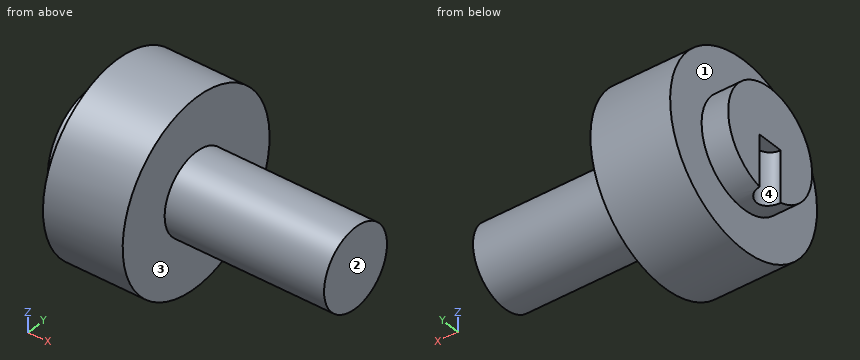
from build123d import *

# Parameters (mm, degrees)
SKETCH_2_R          = 5
CUT_EXTRUDE_1_DEPTH = 20


with BuildPart() as part:
    # Эскиз1 → Повернуть1 (revolve)
    with BuildSketch(Plane.XY, mode=Mode.PRIVATE) as revolve_1_sk:
        Polygon((0, 0), (100, 0), (100, 15), (40, 15), (40, 35), (10, 35), (10, 20), (0, 20), align=None)
    revolve(revolve_1_sk.sketch.rotate(Axis((0, 0, 0), (1, 0, 0)), 90), axis=Axis((0, 0, 0), (1, 0, 0)))

    # Эскиз2 → Вырез-Вытянуть1 (cut)
    with BuildSketch(Plane.XY):
        Circle(SKETCH_2_R)
    extrude(amount=-CUT_EXTRUDE_1_DEPTH, mode=Mode.SUBTRACT)


solid = part.part
CAD build for the part. Positions are in the model's coordinates, mm. Face numbers are marked on the shaded views. A direction names the side the tool comes from. Give positions to 0.01 mm unless a question says otherwise; leave off trailing zeros. Order: outer loops, then holes, each group sorted by start corner. A loop starts at its lowest first (then second) coordinate and runs counter-clockwise, first axis right, second up. Notation, with made-up numbers: (-17, 76) - (36, 76) arc R12 cw to (36, 99) - close; hole circle Ø2 at (63.25, -9.5). An arc over 180 degrees is marked (long way). Write each question's results on one line, items separated by ' | '.
1. Saw through at C-C on x = 25. List the corners of the cut face in (y, z), and give its area (3 significant figures).
Calculated:
outline: circle Ø70 at (0, 0) | area: 3,850 mm2
2. Pin check, flat tips, straight feed: pin 1 (5 mm diameter, centred on y = -27.5, z = -19, fed in from -X); pin 2 (5.5 mm diameter, centred on x = 2, y = 1.5, fed in from -Z); pin 3 (8 mm diameter, centred on x = 33.5, z = 21, fed in from +Y). Stop position of each tip, or through.
Calculated:
pin 1: stops at x = 10 | pin 2: stops at z = -19.94 | pin 3: stops at y = 30.59
3. Saw through at A-A on y = 0. List the corners of the cut face in (x, z).
Calculated:
outline: (0, 0) - (5, 0) - (5, -20) - (10, -20) - (10, -35) - (40, -35) - (40, -15) - (100, -15) - (100, 15) - (40, 15) - (40, 35) - (10, 35) - (10, 20) - (0, 20) - close
4. Saw through at B-B on z = -12. List the corners of the cut face in (x, y), and give its area (3 significant figures).
Calculated:
outline: (0, -16) - (10, -16) - (10, -32.88) - (40, -32.88) - (40, -9) - (100, -9) - (100, 9) - (40, 9) - (40, 32.88) - (10, 32.88) - (10, 16) - (0, 16) - (0, 5) arc R5 cw to (0, -5) - close | area: 3,330 mm2
5. Probe L1, parallel to X at y = -18.5, z = 14; L2, parallel to X at y = -10, z = -12; L3, parallel to Z at x = 57, y = 5.5. List the from-to ranges inside material, lowest first. Write a range as from..to.
Calculated:
L1: x = 10..40 | L2: x = 0..40 | L3: z = -13.96..13.96
6. Saw through at D-D on y = -11. List the corners of the cut face in (x, z), and give its area (3 significant figures).
Calculated:
outline: (0, -16.7) - (10, -16.7) - (10, -33.23) - (40, -33.23) - (40, -10.2) - (100, -10.2) - (100, 10.2) - (40, 10.2) - (40, 33.23) - (10, 33.23) - (10, 16.7) - (0, 16.7) - close | area: 3,550 mm2
7. 3-axis set-ups, long thin cutter, end or side, ignore diameter. For the marked faces 1, 2, 3 and 4: which of +Z, -Z, +X, -X, +Y, -Y reach the whole face in a straight line?
Calculated:
face 1: -X | face 2: +Z, -Z, +X, +Y, -Y | face 3: +X | face 4: -Z, -X
